from build123d import *

# Parameters (mm, degrees)
SKETCH1_R           = 16.192287761
BOSS_EXTRUDE1_DEPTH = 12.7
CUT_EXTRUDE1_DEPTH  = 12.7
FILLET1_R           = 0.809614388
CIRPATTERN1_DEPTH   = 12.7
SKETCH3_R           = 3.175
BOSS_EXTRUDE2_DEPTH = 6.35
SKETCH5_R           = 3.302
BOSS_EXTRUDE3_DEPTH = 3.175


# Read off the part's stored shape, not the designer's step: CirPattern1
with BuildPart() as part:
    # Sketch1 → Boss-Extrude1 (new body)
    with BuildSketch(Plane.XY):
        Circle(SKETCH1_R)
    extrude(amount=BOSS_EXTRUDE1_DEPTH)

    # Sketch2 → Cut-Extrude1 (cut)
    with BuildSketch(Plane.XY.offset(12.7)):
        with BuildLine():
            ThreePointArc((-0.648981162, 9.693672643), (-2.761211409, 13.995350311), (-7.286822608, 15.571672188))
            ThreePointArc((-7.286822608, 15.571672188), (0, 17.192287761), (7.286822608, 15.571672188))
            ThreePointArc((7.286822608, 15.571672188), (2.761211409, 13.995350311), (0.648981162, 9.693672643))
            ThreePointArc((0.648981162, 9.693672643), (0, 9.715372656), (-0.648981162, 9.693672643))
        make_face()
    extrude(amount=-CUT_EXTRUDE1_DEPTH, mode=Mode.SUBTRACT)

    # Fillet1
    # the kernel refuses this fillet: 0.809614388 mm, written as the material it adds along each edge
    with BuildSketch(Plane(origin=(0.648981162, 9.693672643, 12.7), x_dir=(0.12156320456415769, 0.9925836928421162, 0), z_dir=(0, 0, -1))) as fillet1_piece_1:
        with BuildLine():
            CenterArc((0.738327126, -0.808389468), FILLET1_R, 93.152151787, 79.518968538)
            ThreePointArc((-0.064672931, -0.705111371), (-0.025910634, -0.353145064), (0, 0))
            ThreePointArc((0, 0), (0.346904155, -0.009544948), (0.69380831, 0))
        make_face()
    extrude(amount=12.7)
    with BuildSketch(Plane(origin=(-0.648981162, 9.693672643, 12.7), x_dir=(0.9995379445948291, 0.030395679218338256, 0), z_dir=(0, 0, -1))) as fillet1_piece_2:
        with BuildLine():
            CenterArc((0.737574027, -0.809076654), FILLET1_R, 92.088363944, 79.518968538)
            ThreePointArc((-0.063370217, -0.690908233), (-0.022180058, -0.346325921), (0, 0))
            ThreePointArc((0, 0), (0.354035533, -0.006452804), (0.708071066, 0))
        make_face()
    extrude(amount=12.7)
    # the kernel refuses this fillet: 0.809614388 mm, written as the material it takes off along each edge
    with BuildSketch(Plane(origin=(-5.198948894, 15.334963753, 13.415202102), x_dir=(-0.9443027648777296, -0.32907793642885796, 0), z_dir=(0, 0, -1))) as fillet1_2_piece_1:
        with BuildLine():
            CenterArc((0.267182003, -0.809585402), FILLET1_R, 89.515166978, 38.350588161)
            ThreePointArc((-0.229770211, -0.170434439), (-0.115851307, -0.08391464), (0, 0))
            ThreePointArc((0, 0), (0.137016412, 0.000579715), (0.274032824, 0))
        make_face()
    extrude(amount=14.130404205, mode=Mode.SUBTRACT)
    with BuildSketch(Plane(origin=(5.198948894, 15.334963753, 13.415202102), x_dir=(0.9443027648777299, -0.32907793642885697, 0), z_dir=(0, 0, -1))) as fillet1_2_piece_2:
        with BuildLine():
            CenterArc((0.267182003, 0.809585402), FILLET1_R, 232.134244861, 38.350588161)
            ThreePointArc((-0.229770211, 0.170434439), (-0.115851307, 0.08391464), (0, 0))
            ThreePointArc((0, 0), (0.137016412, -0.000579715), (0.274032824, 0))
        make_face()
    extrude(amount=14.130404205, mode=Mode.SUBTRACT)

    # CirPattern1 outline → CirPattern1 (cut)
    with BuildSketch(Plane.XY):
        with BuildLine():
            ThreePointArc((4.958837242, 15.259978898), (6.118325298, 12.120958043), (5.50931312, 8.830522108))
            ThreePointArc((5.50931312, 8.830522108), (5.445351284, 8.311585796), (5.711912975, 7.86177375))
            ThreePointArc((5.711912975, 7.86177375), (6.222081746, 7.747258083), (6.695854212, 7.968449544))
            ThreePointArc((6.695854212, 7.968449544), (9.637377118, 9.564531404), (12.981378188, 9.431523325))
            ThreePointArc((12.981378188, 9.431523325), (12.074523228, 6.21008756), (9.647578607, 3.905749452))
            ThreePointArc((9.647578607, 3.905749452), (9.290809283, 3.523516981), (9.242069335, 3.002930361))
            ThreePointArc((9.242069335, 3.002930361), (9.58749392, 2.610415561), (10.100796975, 2.510886743))
            ThreePointArc((10.100796975, 2.510886743), (13.418692374, 2.073160309), (16.045865882, 0))
            ThreePointArc((16.045865882, 0), (13.418692374, -2.073160309), (10.100796975, -2.510886743))
            ThreePointArc((10.100796975, -2.510886743), (9.58749392, -2.610415561), (9.242069335, -3.002930361))
            ThreePointArc((9.242069335, -3.002930361), (9.290809283, -3.523516981), (9.647578607, -3.905749452))
            ThreePointArc((9.647578607, -3.905749452), (12.074523228, -6.21008756), (12.981378188, -9.431523325))
            ThreePointArc((12.981378188, -9.431523325), (9.637377118, -9.564531404), (6.695854212, -7.968449544))
            ThreePointArc((6.695854212, -7.968449544), (6.222081746, -7.747258083), (5.711912975, -7.86177375))
            ThreePointArc((5.711912975, -7.86177375), (5.445351284, -8.311585796), (5.50931312, -8.830522108))
            ThreePointArc((5.50931312, -8.830522108), (6.118296607, -12.121293054), (4.958445247, -15.260525306))
            ThreePointArc((4.958445247, -15.260525306), (2.174911365, -13.402576589), (0.733322724, -10.382335457))
            ThreePointArc((0.733322724, -10.382335457), (0.480045825, -9.924911338), (0, -9.717686779))
            ThreePointArc((0, -9.717686779), (-0.480045825, -9.924911338), (-0.733322724, -10.382335457))
            ThreePointArc((-0.733322724, -10.382335457), (-2.174911365, -13.402576589), (-4.958445247, -15.260525306))
            ThreePointArc((-4.958445247, -15.260525306), (-6.118296607, -12.121293054), (-5.50931312, -8.830522108))
            ThreePointArc((-5.50931312, -8.830522108), (-5.445351284, -8.311585796), (-5.711912975, -7.86177375))
            ThreePointArc((-5.711912975, -7.86177375), (-6.222081746, -7.747258083), (-6.695854212, -7.968449544))
            ThreePointArc((-6.695854212, -7.968449544), (-9.637377118, -9.564531404), (-12.981378188, -9.431523325))
            ThreePointArc((-12.981378188, -9.431523325), (-12.074523228, -6.21008756), (-9.647578607, -3.905749452))
            ThreePointArc((-9.647578607, -3.905749452), (-9.290809283, -3.523516981), (-9.242069335, -3.002930361))
            ThreePointArc((-9.242069335, -3.002930361), (-9.58749392, -2.610415561), (-10.100796975, -2.510886743))
            ThreePointArc((-10.100796975, -2.510886743), (-13.418692374, -2.073160309), (-16.045865882, 0))
            ThreePointArc((-16.045865882, 0), (-13.418692374, 2.073160309), (-10.100796975, 2.510886743))
            ThreePointArc((-10.100796975, 2.510886743), (-9.58749392, 2.610415561), (-9.242069335, 3.002930361))
            ThreePointArc((-9.242069335, 3.002930361), (-9.290809283, 3.523516981), (-9.647578607, 3.905749452))
            ThreePointArc((-9.647578607, 3.905749452), (-12.074523228, 6.21008756), (-12.981378188, 9.431523325))
            ThreePointArc((-12.981378188, 9.431523325), (-9.637377118, 9.564531404), (-6.695854212, 7.968449544))
            ThreePointArc((-6.695854212, 7.968449544), (-6.222081746, 7.747258083), (-5.711912975, 7.86177375))
            ThreePointArc((-5.711912975, 7.86177375), (-5.445351284, 8.311585796), (-5.50931312, 8.830522108))
            ThreePointArc((-5.50931312, 8.830522108), (-6.118325298, 12.120958043), (-4.958837242, 15.259978898))
            ThreePointArc((-4.958837242, 15.259978898), (-5.20947806, 15.291785512), (-5.457718847, 15.244785597))
            ThreePointArc((-5.457718847, 15.244785597), (0, -16.192287761), (5.457718847, 15.244785597))
            ThreePointArc((5.457718847, 15.244785597), (5.20947806, 15.291785512), (4.958837242, 15.259978898))
        make_face()
    extrude(amount=CIRPATTERN1_DEPTH, mode=Mode.SUBTRACT)

    # Sketch3 → Boss-Extrude2 (add)
    with BuildSketch(Plane(origin=(0, 0, 0), x_dir=(-1, 0, 0), z_dir=(0, 0, -1))):
        with Locations(Location((0, 0, 0), (0, 0, 180))):
            Circle(SKETCH3_R)
    extrude(amount=BOSS_EXTRUDE2_DEPTH)

    # Sketch5 → Boss-Extrude3 (add)
    with BuildSketch(Plane.XY.offset(12.7)):
        with BuildLine():
            Line((-14.735919106, 6.35), (-29.21, 6.35))
            ThreePointArc((-29.21, 6.35), (-31.006051224, 5.606051224), (-31.75, 3.81))
            Line((-31.75, 3.81), (-31.75, -3.81))
            ThreePointArc((-31.75, -3.81), (-31.006051224, -5.606051224), (-29.21, -6.35))
            Line((-29.21, -6.35), (-14.735919106, -6.35))
            ThreePointArc((-14.735919106, -6.35), (16.045865882, 0), (-14.735919106, 6.35))
        make_face()
        with Locations((-25.4, 0)):
            Circle(SKETCH5_R, mode=Mode.SUBTRACT)
    extrude(amount=BOSS_EXTRUDE3_DEPTH)


solid = part.part
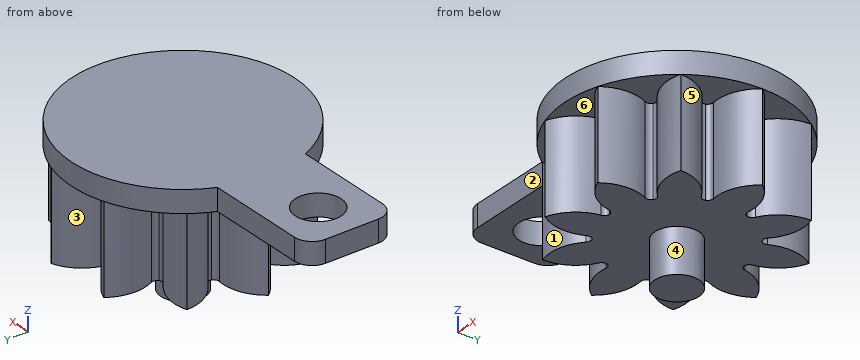
Verification items for the finished model (mm, model axes). Face numbers are marked on the shaded views. A direction names the side the tool comes from. Give positions to 0.01 mm unless a question says otherwise; leave off trailing zeros. Loops run counter-clockwise (first coordinate to the right, second up) from the corner with the lowest first, then second, coordinate; pieces in that order, holes last. Notation, with made-up numbers: (72.25, -27) - (108.25, -27) arc R6 ccw to (108.25, -22) - close; hole circle Ø1 at (34.25, 2). An arc over 180 degrees is marked (long way). Write item = value, one per line. Start each with the question number.
Q1. Cross-section at C-C, the plane y = -0.5. Enter the section's corners in (x, z) (3 decimals).
Q2. Thickness scan on line 1 (Y direction, x = -25.4, z = 14); line 2 (X direction, y = -12, z = 0.5); line 3 (Z direction, x = 1, y = 4.5) (3 decimals). Record the ranges inside material, lowest first.
Q3. Tool access check on the marked faces 1, 2 and 3. Record the directions out of +Z, -Z, +X, -X, +Y, -Y that give a thin tool (end or side, any length) a straight path to the whole face; none if there is none.
Q4. Cross-section at A-A, the plane x = -25.4. Enter the section's corners in (y, z) (3 decimals).
Q5. Mould release check, pull along X, two halves, no side actions. Record for the marked faces 4, 5 and 6: released by +X, released by -X, zero draft, split by the parting line, or undercut.
Q6. Cross-section at D-D, the plane z = -0.75. Enter the section's corners in (x, y) (3 decimals), and give its area (3 significant figures).
Q7. Cross-section at B-B, the plane z = 14. Enter the section's corners in (x, y).
Q8. Depth check by flat-ended pin: P1, Ø2, axis at x = 1.5, y = 9.5, coming from the -Z side; P2, Ø3.5, axis at x = -22.5, z = 15, coming from the +Y side; P3, Ø2, axis at x = 14, y = -4, coming from the -Z side; P4, Ø8.5, axis at x = -25.4, y = 0, coming from the +Z side (3 decimals). Enter the tip coordinate at first touch or a pass-through.
Answer key:
q1.outline = (-31.75, 12.7) - (-28.664, 12.7) - (-28.664, 15.875) - (-31.75, 15.875) - close; (-22.136, 12.7) - (-15.637, 12.7) - (-15.637, 0) - (-3.135, 0) - (-3.135, -6.35) - (3.135, -6.35) - (3.135, 0) - (15.637, 0) - (15.637, 12.7) - (16.038, 12.7) - (16.038, 15.875) - (-22.136, 15.875) - close
q2.line_1 = -6.35 to -3.3, 3.3 to 6.35
q2.line_2 = -6.13 to -1.26, 1.26 to 6.13
q2.line_3 = 0 to 15.875
q3.face_1 = -Z, -Y
q3.face_2 = +Z, -Z, -X, -Y
q3.face_3 = -Z, +Y
q4.outline = (-6.35, 12.7) - (-3.302, 12.7) - (-3.302, 15.875) - (-6.35, 15.875) - close; (3.302, 12.7) - (6.35, 12.7) - (6.35, 15.875) - (3.302, 15.875) - close
q5.face_4 = split by the parting line
q5.face_5 = released by +X
q5.face_6 = undercut
q6.outline = circle Ø6.35 at (0, 0)
q6.area = 31.7 mm^2
q7.outline = (-31.75, -3.81) arc R2.54 ccw to (-29.21, -6.35) - (-14.74, -6.35) arc R16.05 ccw (long way) to (-14.74, 6.35) - (-29.21, 6.35) arc R2.54 ccw to (-31.75, 3.81) - close; hole circle Ø6.6 at (-25.4, 0)
q8.P1 = 0
q8.P2 = 6.35
q8.P3 = 12.7
q8.P4 = 15.875
